Check sheet for the drawn part. Datum: minimum x, y, z corner. Units: mm. A direction names the side the tool comes from. Round coordinates to 2 decimals unless told otherwise and drop trailing zeros. Write each loop counter-clockwise with the first axis right and the second up, starting at its lowest first coordinate (ties: lowest second). Pieces come first, ordered by that corner, then holes. Notation, with made-up numbers: (83, 29) - (126, 29) arc R18 ccw to (126, 37) - close; hole circle Ø9 at (10.5, -40). An arc over 180 degrees is marked (long way). Answer as a JSON object with one key per item and string values. Group by question number.
1) Thickness scan on line 1 (Y direction, x = 76.2, z = 2.1) (3 decimals); line 2 (Z direction, x = 103, y = 30) (3 decimals). Record the ranges inside material, lowest first.
2) Section check D-D (x = 65). Enter the section's corners in (y, z) (3 decimals), then the cut area to 3 significant figures.
3) Set-up check for the marked faces 1 and 2: record each of +Z, -Z, +X, -X, +Y, -Y from which the full face is reachable in a straight line by a thin tool's end or side.
4) Mould release check, pull along Z, two halves, no side actions. Record for the marked faces 3, 4 and 5: +Z half, -Z half, draft (parallel to the pull), parting line (faces both ways), or undercut.
5) Section check C-C (x = 127). Enter the section's corners in (y, z) (3 decimals), then the cut area to 3 significant figures.
6) Section check A-A (z = 31.5). Enter the section's corners in (x, y) (3 decimals).
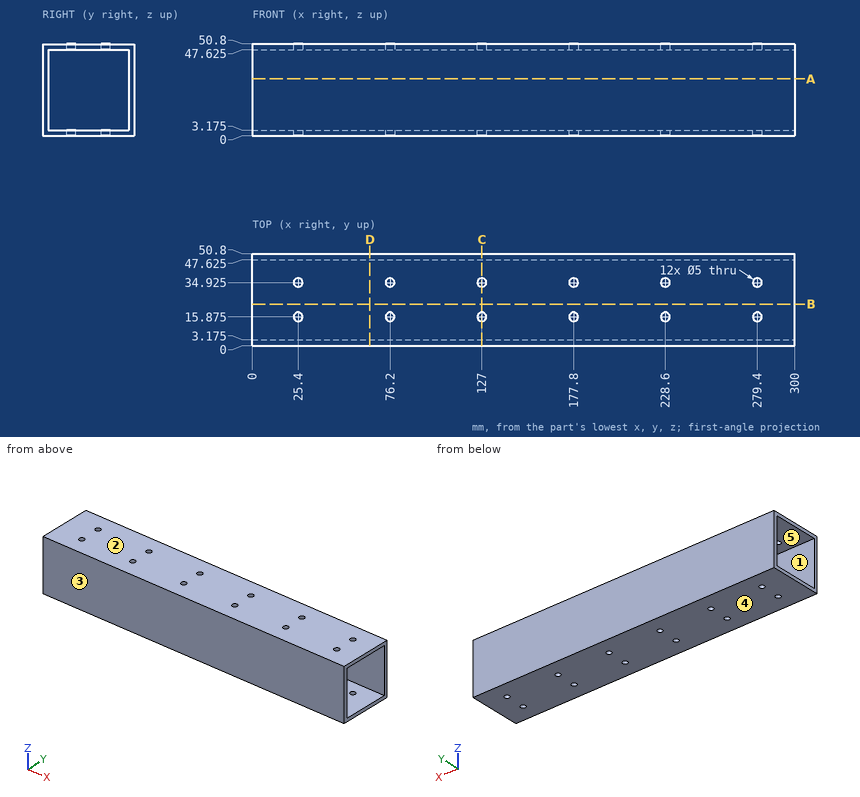
Returned:
{
 "1": {"line 1": "0 to 13.375, 18.375 to 32.425, 37.425 to 50.8", "line 2": "0 to 3.175, 47.625 to 50.8"},
 "2": {"outline": "(0, 0) - (50.8, 0) - (50.8, 50.8) - (0, 50.8) - close; hole (3.175, 3.175) - (47.625, 3.175) - (47.625, 47.625) - (3.175, 47.625) - close", "area": "605 mm2"},
 "3": {"face 1": "+X, -X", "face 2": "+Z, +X, -X, +Y, -Y"},
 "4": {"face 3": "draft", "face 4": "-Z half", "face 5": "undercut"},
 "5": {"outline": "(0, 0) - (13.375, 0) - (13.375, 3.175) - (3.175, 3.175) - (3.175, 47.625) - (13.375, 47.625) - (13.375, 50.8) - (0, 50.8) - close; (18.375, 0) - (32.425, 0) - (32.425, 3.175) - (18.375, 3.175) - close; (18.375, 47.625) - (32.425, 47.625) - (32.425, 50.8) - (18.375, 50.8) - close; (37.425, 0) - (50.8, 0) - (50.8, 50.8) - (37.425, 50.8) - (37.425, 47.625) - (47.625, 47.625) - (47.625, 3.175) - (37.425, 3.175) - close", "area": "541 mm2"},
 "6": {"outline": "(0, 0) - (300, 0) - (300, 3.175) - (0, 3.175) - close; (0, 47.625) - (300, 47.625) - (300, 50.8) - (0, 50.8) - close"}
}
